from build123d import *
from build123d.topology import SkipClean

# Parameters (mm, degrees)
EXTRUDE_1_DEPTH          = 39
SKETCH_2_W               = 3
SKETCH_2_H               = 29
CUT_EXTRUDE_1_DEPTH      = 57.00892786
CUT_EXTRUDE_2_DEPTH      = 57.187187152
CUT_EXTRUDE_2_DEPTH_BACK = 57.187187152
EXTRUDE_START            = 3
SKETCH_4_R               = 3
EXTRUDE_2_DEPTH          = 3
HOLE_WIZARD_M3_1_REACH   = 88.522
HOLE_WIZARD_M3_1_BORE_R  = 1.25
HOLE_WIZARD_M2_5_1_D     = 2.05
CHAMFER_1_SIZE           = 0.5
SKETCH_10_W              = 4
SKETCH_10_H              = 70
SKETCH_10_W_2            = 66
SKETCH_10_H_2            = 4
EXTRUDE_1_2_DEPTH        = 2
FILLET_1_R               = 1


with BuildPart() as part:
    # Sketch 1 → Extrude 1 (new, symmetric)
    with BuildSketch(Plane.XY):
        Polygon((-40, 0), (-40, 2), (-37, 2), (-37, 6), (-33, 6), (-33, 2), (33, 2), (33, 6), (37, 6), (37, 2), (40, 2), (40, 0), align=None)
    extrude(amount=EXTRUDE_1_DEPTH, both=True)

    # Sketch 2 → Cut-Extrude 1 (cut, through all)
    with BuildSketch(Plane(origin=(0, 2, 0), x_dir=(1, 0, 0), z_dir=(0, 1, 0))):
        with Locations((-38.5, 24.5)):
            Rectangle(SKETCH_2_W, SKETCH_2_H)
        with BuildLine():
            Line((-24.171572875, -35), (24.171572875, -35))
            ThreePointArc((24.171572875, -35), (25.267949192, -33.550510257), (27, -33))
            Line((27, -33), (33, -33))
            Line((33, -33), (33, 33))
            Line((33, 33), (27, 33))
            ThreePointArc((27, 33), (25.267949192, 33.550510257), (24.171572875, 35))
            Line((24.171572875, 35), (-24.171572875, 35))
            ThreePointArc((-24.171572875, 35), (-25.267949192, 33.550510257), (-27, 33))
            Line((-27, 33), (-33, 33))
            Line((-33, 33), (-33, -33))
            Line((-33, -33), (-27, -33))
            ThreePointArc((-27, -33), (-25.267949192, -33.550510257), (-24.171572875, -35))
        make_face()
        with Locations((-38.5, -24.5)):
            Rectangle(SKETCH_2_W, SKETCH_2_H)
        with Locations((38.5, -24.5)):
            Rectangle(SKETCH_2_W, SKETCH_2_H)
        with Locations((38.5, 24.5)):
            Rectangle(SKETCH_2_W, SKETCH_2_H)
    extrude(amount=-CUT_EXTRUDE_1_DEPTH, mode=Mode.SUBTRACT)

    # Sketch 3 → Cut-Extrude 2 (cut, two sides: drawn at the far end of the back side and taken through both)
    with BuildSketch(Plane(origin=(0, 0, 0), x_dir=(0, 0, -1), z_dir=(1, 0, 0)).offset(-CUT_EXTRUDE_2_DEPTH_BACK)):
        with BuildLine():
            Line((-22, 2), (22, 2))
            Line((22, 2), (22, 3))
            ThreePointArc((22, 3), (25, 6), (28, 3))
            Line((28, 3), (28, 2))
            Line((28, 2), (39, 2))
            Line((39, 2), (39, 7))
            Line((39, 7), (-39, 7))
            Line((-39, 7), (-39, 2))
            Line((-39, 2), (-28, 2))
            Line((-28, 2), (-28, 3))
            ThreePointArc((-28, 3), (-25, 6), (-22, 3))
            Line((-22, 3), (-22, 2))
        make_face()
    extrude(amount=CUT_EXTRUDE_2_DEPTH + CUT_EXTRUDE_2_DEPTH_BACK, mode=Mode.SUBTRACT)

    # Sketch 4 → Extrude 2 (add)
    with SkipClean():  # the faces are left unmerged after this step: merging them gives an invalid solid
        with BuildSketch(Plane(origin=(0, 2, 0), x_dir=(1, 0, 0), z_dir=(0, 1, 0)).offset(EXTRUDE_START)):
            with Locations(Location((-27, 36, 0), (0, 0, 270))):
                Circle(SKETCH_4_R)
            with Locations(Location((-27, -36, 0), (0, 0, 90))):
                Circle(SKETCH_4_R)
            with Locations(Location((27, -36, 0), (0, 0, 270))):
                Circle(SKETCH_4_R)
            with Locations(Location((27, 36, 0), (0, 0, 90))):
                Circle(SKETCH_4_R)
        extrude(amount=-EXTRUDE_2_DEPTH)

    # Hole Wizard M3 _1 bore → Hole Wizard M3 _1 (cut, up to next)
    with BuildSketch(Plane.ZY.offset(37), mode=Mode.PRIVATE) as hole_wizard_m3_1_sk1:
        with Locations((-25, 3)):
            Circle(HOLE_WIZARD_M3_1_BORE_R)
    hole_wizard_m3_1_tool1 = extrude(hole_wizard_m3_1_sk1.sketch, amount=-HOLE_WIZARD_M3_1_REACH, mode=Mode.PRIVATE) & part.part
    # Hole Wizard M3 _1 bore → Hole Wizard M3 _1 (cut, up to next)
    with BuildSketch(Plane.ZY.offset(37), mode=Mode.PRIVATE) as hole_wizard_m3_1_sk2:
        with Locations((25, 3)):
            Circle(HOLE_WIZARD_M3_1_BORE_R)
    hole_wizard_m3_1_tool2 = extrude(hole_wizard_m3_1_sk2.sketch, amount=-HOLE_WIZARD_M3_1_REACH, mode=Mode.PRIVATE) & part.part
    hole_wizard_m3_1_1 = hole_wizard_m3_1_tool1.solids().sort_by_distance((-37, 3, -25))[0]
    add(hole_wizard_m3_1_1, mode=Mode.SUBTRACT)
    hole_wizard_m3_1_2 = hole_wizard_m3_1_tool2.solids().sort_by_distance((-37, 3, 25))[0]
    add(hole_wizard_m3_1_2, mode=Mode.SUBTRACT)
    hole_wizard_m3_1 = hole_wizard_m3_1_1 + hole_wizard_m3_1_2  # Hole Wizard M3 _1 as one shape, for the pattern or mirror that repeats it

    # Hole Wizard M2.5 _1 (through all)
    with Locations(Plane(origin=(0, 5, 0), x_dir=(1, 0, 0), z_dir=(0, 1, 0))):
        with Locations((-27, 36), (27, 36), (-27, -36), (27, -36)):
            Hole(HOLE_WIZARD_M2_5_1_D / 2)

    # Mirror 1: Hole Wizard M3 _1 across plane
    add(hole_wizard_m3_1.mirror(Plane(origin=(0, 0, 0), x_dir=(0, 0, 1), z_dir=(1, 0, 0))), mode=Mode.SUBTRACT)

    # Chamfer 1
    chamfer_1_edges = [part.edges().sort_by_distance(p)[0] for p in [
        (33, 2.5, -28),
        (-33, 2.5, -28),
        (33, 6, -25),
        (-33, 6, -25),
        (33, 2.5, -22),
        (-33, 2.5, -22),
        (33, 2.5, 22),
        (-33, 2.5, 22),
        (33, 6, 25),
        (-33, 6, 25),
        (33, 2.5, 28),
        (-33, 2.5, 28),
        (40, 1, -10),
        (40, 1, 10),
        (-40, 1, -10),
        (-40, 1, 10),
    ]]
    chamfer(chamfer_1_edges, length=CHAMFER_1_SIZE)

    # Sketch 10 → Extrude 1 2 (add)
    with BuildSketch(Plane(origin=(0, 2, 0), x_dir=(1, 0, 0), z_dir=(0, 1, 0))):
        with Locations((-15, 0)):
            Rectangle(SKETCH_10_W, SKETCH_10_H)
        with Locations((0, 12.5)):
            Rectangle(SKETCH_10_W_2, SKETCH_10_H_2)
        with Locations((0, -12.5)):
            Rectangle(SKETCH_10_W_2, SKETCH_10_H_2)
        with Locations((15, 0)):
            Rectangle(SKETCH_10_W, SKETCH_10_H)
    extrude(amount=-EXTRUDE_1_2_DEPTH)

    # Fillet 1
    fillet_1_edges = [part.edges().sort_by_distance(p)[0] for p in [
        (37, 1, 39),
        (-37, 1, -39),
        (-37, 1, 39),
        (37, 1, -39),
        (-13, 1, -35),
        (-13, 1, -10.5),
        (-17, 1, -14.5),
        (-17, 1, 10.5),
        (-13, 1, 35),
        (-13, 1, 14.5),
        (-17, 1, -35),
        (-17, 1, 35),
        (-33, 1, 14.5),
        (-33, 1, 10.5),
        (-17, 1, 14.5),
        (-33, 1, -10.5),
        (-17, 1, -10.5),
        (-33, 1, -14.5),
        (-13, 1, -14.5),
        (13, 1, -14.5),
        (-13, 1, 10.5),
        (13, 1, 10.5),
        (17, 1, -10.5),
        (33, 1, -10.5),
        (33, 1, -14.5),
        (13, 1, 14.5),
        (13, 1, 35),
        (17, 1, 35),
        (17, 1, 14.5),
        (33, 1, 14.5),
        (33, 1, 10.5),
        (13, 1, -10.5),
        (17, 1, 10.5),
        (17, 1, -14.5),
        (17, 1, -35),
        (13, 1, -35),
        (-24.171572875, 1, 35),
        (-33, 1, 33),
        (-33, 1, -33),
        (-24.171572875, 1, -35),
        (24.171572875, 1, -35),
        (33, 1, -33),
        (33, 1, 33),
        (24.171572875, 1, 35),
    ]]
    fillet(fillet_1_edges, radius=FILLET_1_R)


solid = part.part
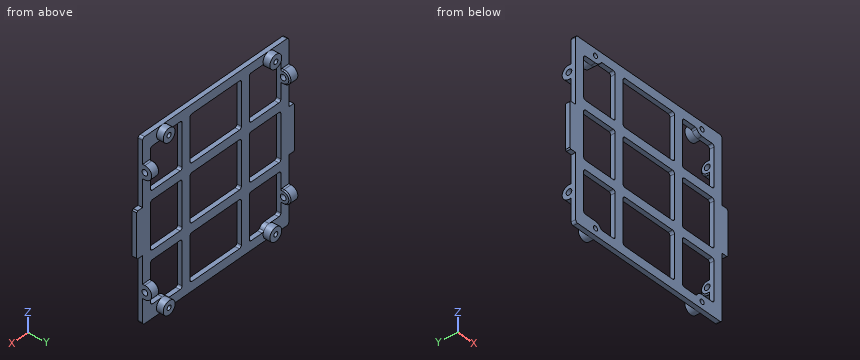
The model under review builds one solid part; all positions refer to its coordinate system, in mm. Give positions to 0.01 mm unless a question says otherwise; leave off trailing zeros. Order: outer loops, then holes, each group sorted by start corner. A loop starts at its lowest first (then second) coordinate and runs counter-clockwise, first axis right, second up. Notation, with made-up numbers: (28.5, 79.5) -> (77.5, 79.5) arc R29 ccw to (77.5, 114.5) -> close; hole circle Ø9 at (60, -16.75). An arc over 180 degrees is marked (long way). Write item = value, one per line. Start each with the question number.
(1) Take a section at C-C (z = -6). Write out the cut boundary in (x, y).
(2) Take a section at A-A (z = 36). Write out the cut boundary in (x, y) (3 decimals), plus the area to 4 significant figures.
(3) For pin 1 Ø1.5 at (x, z) = (0.5, 8) entering from +Y; pin 2 Ø1.6 at (y, z) = (1.5, -24) entering from +X; pin 3 Ø0.6 at (y, z) = (1, 27.5) entering from -X; pin 4 Ø0.8 at (x, y) = (35, 2.5) entering from -Z, all flat-tipped, find the tip position at first contact; note any pin that passes through.
(4) Take a section at B-B (x = 1.5). Write out the cut boundary in (y, z), plus the area to 3 significant figures.
(5) For L1, parallel to X at y = 0.55, z = 27; L2, parallel to Z at x = -2.5, y = 1.1; L3, parallel to Z at x = -25, y = 1.85, list the stretches that pass through material, from the lowest coordinate up. Write a range as from..to.
(6) Take a section at D-D (z = -25). Write out the cut boundary in (x, y), plus the area to 4 significant figures.
Returned:
q1.outline = (-40, 0) -> (-33, 0) -> (-33, 2) -> (-40, 2) -> close; (-17, 0) -> (-13, 0) -> (-13, 2) -> (-17, 2) -> close; (13, 0) -> (17, 0) -> (17, 2) -> (13, 2) -> close; (33, 0) -> (40, 0) -> (40, 2) -> (33, 2) -> close
q2.outline = (-37, 0) -> (-28.025, 0) -> (-28.025, 5) -> (-30, 5) -> (-30, 2) -> (-37, 2) -> close; (-25.975, 0) -> (25.975, 0) -> (25.975, 5) -> (24, 5) -> (24, 2) -> (-24, 2) -> (-24, 5) -> (-25.975, 5) -> close; (28.025, 0) -> (37, 0) -> (37, 2) -> (30, 2) -> (30, 5) -> (28.025, 5) -> close
q2.area = 163.5 mm²
q3.pin_1 = through
q3.pin_2 = 37
q3.pin_3 = -37
q3.pin_4 = -28
q4.outline = (0, -39) -> (2, -39) -> (2, -35) -> (0, -35) -> close; (0, -14.5) -> (2, -14.5) -> (2, -10.5) -> (0, -10.5) -> close; (0, 10.5) -> (2, 10.5) -> (2, 14.5) -> (0, 14.5) -> close; (0, 35) -> (2, 35) -> (2, 39) -> (0, 39) -> close
q4.area = 32.0 mm²
q5.L1 = -37..-33, -17..-13, 13..17, 33..37
q5.L2 = -39..-35, -14.5..-10.5, 10.5..14.5, 35..39
q5.L3 = -39..-33.76, -14.5..-10.5, 10.5..14.5, 33.76..39
q6.outline = (-37, 0) -> (-33, 0) -> (-33, 1.75) -> (-37, 1.75) -> close; (-37, 4.25) -> (-33, 4.25) -> (-33, 5.5) -> (-33.5, 6) -> (-37, 6) -> close; (-17, 0) -> (-13, 0) -> (-13, 2) -> (-17, 2) -> close; (13, 0) -> (17, 0) -> (17, 2) -> (13, 2) -> close; (33, 0) -> (37, 0) -> (37, 1.75) -> (33, 1.75) -> close; (33, 4.25) -> (37, 4.25) -> (37, 6) -> (33.5, 6) -> (33, 5.5) -> close
q6.area = 43.75 mm²
